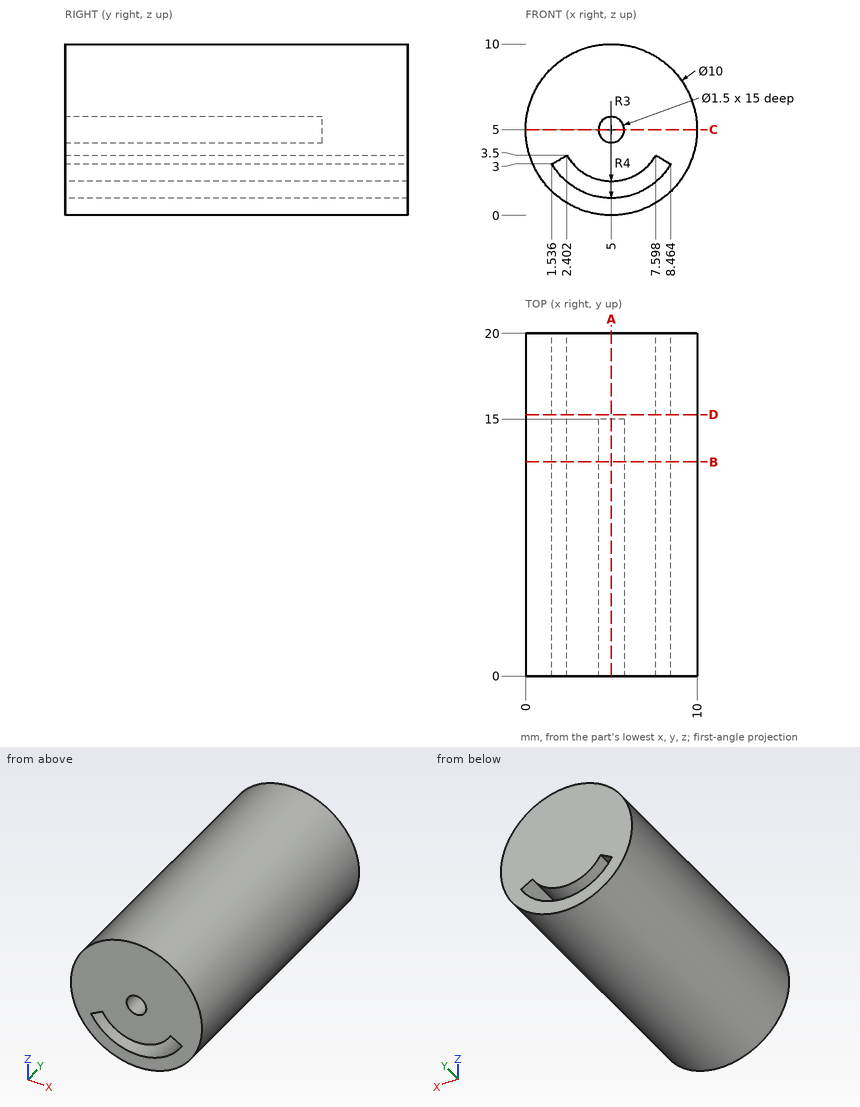
The figure shows three views and two pictorial views of one solid part (mm, origin at its lowest corner). Answer the questions. Coordinates: 2 decimals unless noted, no trailing zeros. Loops run counter-clockwise (first coordinate to the right, second up) from the corner with the lowest first, then second, coordinate; pieces in that order, holes last.
1) Find section A-A on x = 5. Write down the section's boundary in (y, z), then the cut area to 4 significant figures.
2) Find section D-D on y = 15.25. Write down the section's boundary in (x, z), then the cut area to 3 significant figures.
3) Flat-ended cylindrical pins translate along their axes: pin 1 Ø2 at (x, y) = (6.5, 9.5) entering from +Z (3 decimals); pin 2 Ø4 at (x, y) = (8.5, 16.5) entering from +Z; pin 3 Ø2 at (y, z) = (12.5, 6.5) entering from -X (3 decimals). Find the tip coordinate at first contact, or state that the pin passes through.
4) Find section C-C on z = 5. Write down the section's boundary in (x, y).
5) Find section B-B on y = 12.5. Write down the section's boundary in (x, z).
6) Find the intervals of material crossed by L1, parallel to X at y = 10.5, z = 5; L2, parallel to X at y = 17.5, z = 1.5; L3, parallel to Z at x = 8, y = 15.75, in increasing order.
Values:
1. outline: (0, 0) - (20, 0) - (20, 1) - (0, 1) - close; (0, 2) - (20, 2) - (20, 10) - (0, 10) - (0, 5.75) - (15, 5.75) - (15, 4.25) - (0, 4.25) - close
1. area: 157.5 mm2
2. outline: circle Ø10 at (5, 5); hole (1.54, 3) arc R4 ccw to (8.46, 3) - (7.6, 3.5) arc R3 cw to (2.4, 3.5) - close
2. area: 71.2 mm2
3. pin 1: stops at z = 9.975
3. pin 2: stops at z = 9.77
3. pin 3: stops at x = 0.025
4. outline: (0, 0) - (4.25, 0) - (4.25, 15) - (5.75, 15) - (5.75, 0) - (10, 0) - (10, 20) - (0, 20) - close
5. outline: circle Ø10 at (5, 5); hole (1.54, 3) arc R4 ccw to (8.46, 3) - (7.6, 3.5) arc R3 cw to (2.4, 3.5) - close; hole circle Ø1.5 at (5, 5)
6. L1: x = 0 to 4.25, 5.75 to 10
6. L2: x = 1.43 to 3.06, 6.94 to 8.57
6. L3: z = 1 to 2.35, 3.27 to 9
